For this review, use the dimensioned drawing (mm, ordinates from the lowest corner) and the shaded views. Round coordinates to 2 decimals unless told otherwise and drop trailing zeros. Order: outer loops, then holes, each group sorted by start corner. A loop starts at its lowest first (then second) coordinate and runs counter-clockwise, first axis right, second up. Notation, with made-up numbers: (80, 66) -> (136, 66) arc R30 ccw to (136, 94) -> close; hole circle Ø4 at (52.25, -2.5). An arc over 180 degrees is marked (long way). Answer in a Markdown table with one row per item.
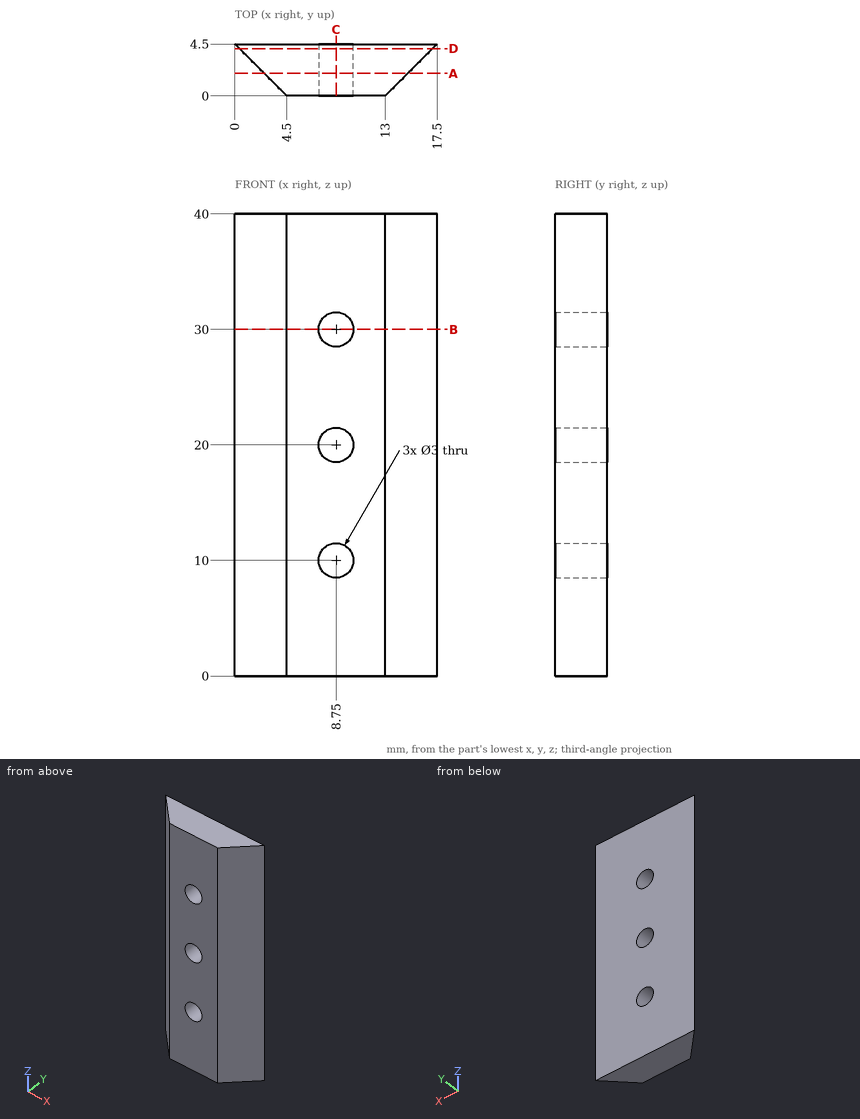
Q1. Take a section at B-B, the plane z = 30. Write out the cut boundary in (x, y).
Answer key:
| item | result |
|---|---|
| outline | (0, 4.5) -> (4.5, 0) -> (7.25, 0) -> (7.25, 4.5) -> close; (10.25, 0) -> (13, 0) -> (17.5, 4.5) -> (10.25, 4.5) -> close |
Q2. Take a section at A-A, the plane y = 1.95. Write out the cut boundary in (x, z), then the cut area to 3 significant figures.
Answer key:
| item | result |
|---|---|
| outline | (2.55, 0) -> (14.95, 0) -> (14.95, 40) -> (2.55, 40) -> close; hole circle Ø3 at (8.75, 10); hole circle Ø3 at (8.75, 20); hole circle Ø3 at (8.75, 30) |
| area | 475 mm^2 |
Q3. To check wall thickness, follow probe 1 along Z at (x, y) = (8.75, 3.5); probe 2 along Z at (x, y) = (10, 3.05); probe 3 along Y at (x, z) = (16, 2). State the ranges of each line that lie inside material, in increasing order.
Answer key:
| item | result |
|---|---|
| probe 1 | z = 0 to 8.5, 11.5 to 18.5, 21.5 to 28.5, 31.5 to 40 |
| probe 2 | z = 0 to 9.17, 10.83 to 19.17, 20.83 to 29.17, 30.83 to 40 |
| probe 3 | y = 3 to 4.5 |
Q4. Take a section at D-D, the plane y = 4.1. Write out the cut boundary in (x, z).
Answer key:
| item | result |
|---|---|
| outline | (0.4, 0) -> (17.1, 0) -> (17.1, 40) -> (0.4, 40) -> close; hole circle Ø3 at (8.75, 10); hole circle Ø3 at (8.75, 20); hole circle Ø3 at (8.75, 30) |
Q5. Take a section at C-C, the plane x = 8.75. Write out the cut boundary in (y, z).
Answer key:
| item | result |
|---|---|
| outline | (0, 0) -> (4.5, 0) -> (4.5, 8.5) -> (0, 8.5) -> close; (0, 11.5) -> (4.5, 11.5) -> (4.5, 18.5) -> (0, 18.5) -> close; (0, 21.5) -> (4.5, 21.5) -> (4.5, 28.5) -> (0, 28.5) -> close; (0, 31.5) -> (4.5, 31.5) -> (4.5, 40) -> (0, 40) -> close |
Q6. Clearance check with flat-ended pins moving along their axes: pin 1 Ø1.5 at (y, z) = (3, 34) entering from +X; pin 2 Ø2 at (y, z) = (1, 22.5) entering from -X; pin 3 Ø1 at (y, z) = (1.5, 12.5) entering from +X. State where each tip first meets the part, or that it passes through.
Answer key:
| item | result |
|---|---|
| pin 1 | stops at x = 16.75 |
| pin 2 | stops at x = 2.5 |
| pin 3 | stops at x = 15 |
